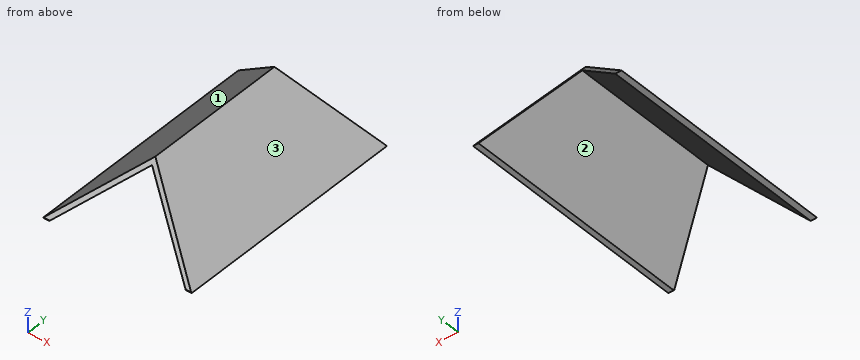
```python
from build123d import *

# Parameters (mm, degrees)
F1_DEPTH      = 203.2
F3_DEPTH      = 124.968
F3_DEPTH_BACK = 110.49
F5_DEPTH      = 83.566
F5_DEPTH_BACK = 103.124


with BuildPart() as f1:
    # F0 (on Front) → F1 (new body)
    with BuildSketch(Plane.XZ):
        Polygon((63.5, -8.2080368082), (0, 50.8), (-63.5, -8.2080368082), (-58.0332870326, -8.2080368082), (0, 45.72), (58.8067129674, -8.2080368082), align=None)
    extrude(amount=F1_DEPTH)

    # F2 (on Right) → F3 (cut, two sides)
    with BuildSketch(Plane.YZ) as f3_sk:
        Polygon((0, -8.2080368082), (0, 51.2279631918), (-40.090088207, 51.2279631918), align=None)
    extrude(amount=-F3_DEPTH, mode=Mode.SUBTRACT)
    extrude(f3_sk.sketch, amount=F3_DEPTH_BACK, mode=Mode.SUBTRACT)

    # F4 (on Right) → F5 (cut, two sides)
    with BuildSketch(Plane.YZ) as f5_sk:
        Polygon((-203.4754604101, 51.2279631918), (-203.4754604101, -8.2080368082), (-163.3853722031, 51.2279631918), align=None)
    extrude(amount=-F5_DEPTH, mode=Mode.SUBTRACT)
    extrude(f5_sk.sketch, amount=F5_DEPTH_BACK, mode=Mode.SUBTRACT)


solid = f1.part
```
Can you work these out from the model? Positions are in its coordinate system, mm. Face numbers are marked on the shaded views. Coordinates: 2 decimals unless noted, no trailing zeros. Loops run counter-clockwise (first coordinate to the right, second up) from the corner with the lowest first, then second, coordinate; pieces in that order, holes last. Notation, with made-up numbers: (58, 3) -> (78, 3) arc R26 cw to (78, 36) -> close; hole circle Ø6 at (47, -25). An arc over 180 degrees is marked (long way). Put each result on its own line as item: value. Start each with the question number.
Q1. I want a section at C-C (y = -45). Write out the boundary of the cut face in (x, z), plus the area to 3 significant figures.
Q2. Thinking about a two-plate mould opening in X: for the marked faces 1, 2 and 3, which applies, pulls with the +X half, pulls with the -X half, needs draft (parallel to the pull), parting line crosses it, or undercut?
Q3. I want a section at B-B (y = -185.5). Write out the boundary of the cut face in (x, z), plus the area to 3 significant figures.
Q4. I want a section at A-A (z = 22). Write out the boundary of the cut face in (x, y), plus the area to 3 significant figures.
Q5. If I drill on line 1 (X direction, y = -144.5, z = 0); line 2 (X direction, y = -156, z = 11.5); line 3 (Z direction, x = 46, y = -13.5), over which ranges is the centre line in solid material (lowest first)? Write a range as [from, to].
Q6. I want a section at D-D (x = 54). Write out the boundary of the cut face in (y, z).
Q7. I'm going to push flat-ended pins straight in: P1, Ø6, axis at y = -52.5, z = 9, coming from the +X side; P2, Ø1.5, axis at x = -44, y = -46.5, coming from the -Z side; P3, Ø10, axis at x = -42.5, z = 11.5, coming from the -Y side. Where does each tip first touch, or does it pass through?
Taken from the geometry:
1. outline: (-63.5, -8.21) -> (-58.03, -8.21) -> (0, 45.72) -> (58.81, -8.21) -> (63.5, -8.21) -> (0, 50.8) -> close
1. area: 597 mm2
2. face 1: pulls with the -X half
2. face 2: undercut
2. face 3: pulls with the +X half
3. outline: (-63.5, -8.21) -> (-58.03, -8.21) -> (-29.35, 18.44) -> (-34.82, 18.44) -> close; (29.75, 18.44) -> (58.81, -8.21) -> (63.5, -8.21) -> (34.82, 18.44) -> close
3. area: 276 mm2
4. outline: (-30.99, -183.1) -> (-25.53, -183.1) -> (-25.53, -20.38) -> (-30.99, -20.38) -> close; (25.87, -183.1) -> (30.99, -183.1) -> (30.99, -20.38) -> (25.87, -20.38) -> close
4. area: 1,720 mm2
5. line 1: x = [-54.67, -49.2], [49.86, 54.67]
5. line 2: x = [-42.29, -36.82], [37.32, 42.29]
5. line 3: z = [3.54, 8.05]
6. outline: (-200.5, -3.8) -> (-2.97, -3.8) -> (-5.95, 0.62) -> (-197.52, 0.62) -> close
7. P1: stops at x = 48.21
7. P2: stops at z = 4.14
7. P3: stops at y = -193.55
